Can you work these out from the model? Positions are in its coordinate system, mm. Face numbers are marked on the shaded views. A direction names the side the tool comes from. Give positions to 0.01 mm unless a question says otherwise; leave off trailing zeros. Order: outer loops, then holes, each group sorted by start corner. A loop starts at its lowest first (then second) coordinate and runs counter-clockwise, first axis right, second up. Notation, with made-up numbers: (42.5, 36) - (59.5, 36) arc R25 ccw to (59.5, 64) - close; hole circle Ø10 at (10, 84.25). An arc over 180 degrees is marked (long way). Answer as CSV lines item,"result".
```python
from build123d import *

# Parameters (mm, degrees)
EXTRUDE_1_DEPTH     = 36
SKETCH_2_R          = 1.75
CUT_EXTRUDE_1_DEPTH = 41.28690122
SKETCH_3_W          = 0.252686492
SKETCH_3_H          = 10
EXTRUDE_2_DEPTH     = 36
SKETCH_4_R          = 2.75
CUT_EXTRUDE_2_DEPTH = 41.286901364
SKETCH_5_W          = 10
SKETCH_5_H          = 36
CUT_EXTRUDE_3_DEPTH = 0.3


with BuildPart() as part:
    # Эскиз1 → Бобышка-Вытянуть1 (new body)
    with BuildSketch(Plane(origin=(0, 0, 0), x_dir=(1, 0, 0), z_dir=(0, 1, 0))):
        with BuildLine():
            Line((-4.558992206, 17.5), (0, 17.5))
            Line((0, 17.5), (0, -17.5))
            Line((0, -17.5), (-4.558992206, -17.5))
            ThreePointArc((-4.558992206, -17.5), (-3, 0), (-4.558992206, 17.5))
        make_face()
    extrude(amount=EXTRUDE_1_DEPTH)

    # Эскиз2 → Вырез-Вытянуть1 (cut, through all)
    with BuildSketch(Plane(origin=(0, 0, 0), x_dir=(0, 0, -1), z_dir=(1, 0, 0))):
        with Locations((-10, 28)):
            Circle(SKETCH_2_R)
        with Locations((10, 28)):
            Circle(SKETCH_2_R)
        with Locations((10, 8)):
            Circle(SKETCH_2_R)
        with Locations((-10, 8)):
            Circle(SKETCH_2_R)
    extrude(amount=-CUT_EXTRUDE_1_DEPTH, mode=Mode.SUBTRACT)

    # Эскиз3 → Бобышка-Вытянуть2 (add, through all)
    with BuildSketch(Plane(origin=(0, 36, 0), x_dir=(1, 0, 0), z_dir=(0, 1, 0))):
        with Locations((-3, 0)):
            Rectangle(SKETCH_3_W, SKETCH_3_H)
    extrude(amount=-EXTRUDE_2_DEPTH)

    # Эскиз4 → Вырез-Вытянуть2 (cut, through all)
    with BuildSketch(Plane(origin=(0, 0, 0), x_dir=(0, 0, -1), z_dir=(1, 0, 0))):
        with Locations((0, 20.5)):
            Circle(SKETCH_4_R)
    extrude(amount=-CUT_EXTRUDE_2_DEPTH, mode=Mode.SUBTRACT)

    # Эскиз5 → Вырез-Вытянуть3 (cut)
    with BuildSketch(Plane.ZY.offset(3.126343246)):
        with Locations((0, 18)):
            Rectangle(SKETCH_5_W, SKETCH_5_H)
    extrude(amount=-CUT_EXTRUDE_3_DEPTH, mode=Mode.SUBTRACT)


solid = part.part
```
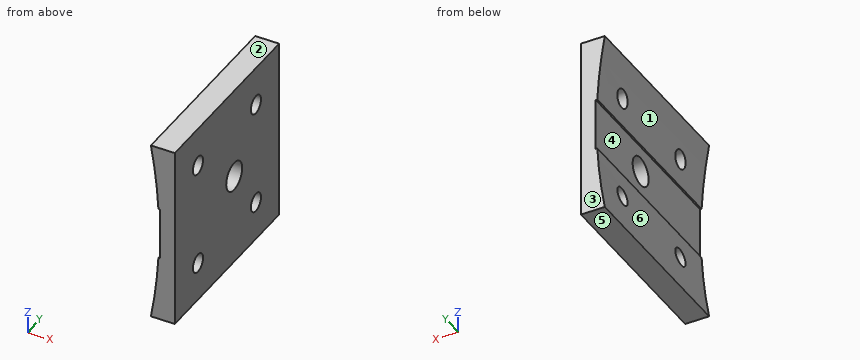
1) I need wall thicknesses on line 1 along Y through (x, z) = (-1.65, 10); line 2 along Z through (x, y) = (-0.9, 8); line 3 along Y through (x, z) = (-1.9, 0). Which ranges of each line are inside material? Lowest first, please. Write a range as [from, to].
Answer block:
line 1,"[0, 6.25], [9.75, 26.25], [29.75, 36]"
line 2,"[-17.5, -11.75], [-8.25, 8.25], [11.75, 17.5]"
line 3,"[0, 17.75], [23.25, 36]"
2) Which directions (+Z, -Z, +X, -X, +Y, -Y) give clear straight access to the entire face, cutting with the end or side of a thin tool? Please do the marked faces 5 and 6.
Answer block:
face 5,"-Z, +X, -X, +Y, -Y"
face 6,"-X, +Y, -Y"
3) If we mould it in two halves opening along Z, with no side actions, what happens to the marked faces 1, 2, 3 and 4? For each: +Z half, -Z half, draft (parallel to the pull), parting line (faces both ways), or undercut.
Answer block:
face 1,"undercut"
face 2,"+Z half"
face 3,"draft"
face 4,"undercut"
4) I want a section at A-A on z = 0. Write out the boundary of the cut face in (x, y), plus the area to 3 significant figures.
Answer block:
outline,"(-2.83, 0) - (0, 0) - (0, 17.75) - (-2.83, 17.75) - close; (-2.83, 23.25) - (0, 23.25) - (0, 36) - (-2.83, 36) - close"
area,"86.2 mm2"
5) I want a section at C-C on y = 20.5. Write out the boundary of the cut face in (x, z).
Answer block:
outline,"(-4.56, -17.5) - (0, -17.5) - (0, -2.75) - (-2.83, -2.75) - (-2.83, -5) - (-3.13, -5) arc R99 cw to start; (-4.56, 17.5) arc R99 cw to (-3.13, 5) - (-2.83, 5) - (-2.83, 2.75) - (0, 2.75) - (0, 17.5) - close"
6) I want a section at B-B on x = -1.55. Write out the boundary of the cut face in (y, z).
Answer block:
outline,"(0, -17.5) - (36, -17.5) - (36, 17.5) - (0, 17.5) - close; hole circle Ø3.5 at (8, -10); hole circle Ø3.5 at (8, 10); hole circle Ø5.5 at (20.5, 0); hole circle Ø3.5 at (28, -10); hole circle Ø3.5 at (28, 10)"
7) I want a section at D-D on z = 10. Write out the boundary of the cut face in (x, y), plus the area to 3 significant figures.
Answer block:
outline,"(-3.51, 0) - (0, 0) - (0, 6.25) - (-3.51, 6.25) - close; (-3.51, 9.75) - (0, 9.75) - (0, 26.25) - (-3.51, 26.25) - close; (-3.51, 29.75) - (0, 29.75) - (0, 36) - (-3.51, 36) - close"
area,"102 mm2"
8) I'm going to push flat-ended pins straight in: P1, Ø2, axis at y = 9.5, z = 11, coming from the -X side; P2, Ø5, axis at y = 14, z = -6.5, coming from the -X side; P3, Ø3, axis at y = 8, z = -10, coming from the +X side; P4, Ø11, axis at y = 20, z = -1.5, coming from the -X side. Where does each tip first touch, or does it pass through?
Answer block:
P1,"x = -3.73"
P2,"x = -3.41"
P3,"through"
P4,"x = -3.25"
